Here's the drawing with two shaded views (mm, measured from the low corner). I have some questions. A direction names the side the tool comes from. Coordinates: 2 decimals unless noted, no trailing zeros. Order: outer loops, then holes, each group sorted by start corner. A loop starts at its lowest first (then second) coordinate and runs counter-clockwise, first axis right, second up. Notation, with made-up numbers: (-11.75, 23.25) -> (46.25, 23.25) arc R13 ccw to (46.25, 28.25) -> close; hole circle Ø8 at (86, -10.5). An arc over 180 degrees is marked (long way). Answer in a Markdown table with one row per item. Add a question column.
1. On a 3-axis mill with a long thin cutter (end or side, diameter ignored), from which of +Z, -Z, +X, -X, +Y, -Y can I reach the whole of each face in a straight line? I mean the marked faces 1 and 2. Say none if no direction works.
2. Imagine slicing it at D-D on y = 17. Write out the boundary of the cut face in (x, z).
3. Imagine slicing it at A-A on y = 10. Write out the boundary of the cut face in (x, z), plus the area to 3 significant figures.
4. Imagine slicing it at B-B on x = 10. Write out the boundary of the cut face in (y, z), plus the area to 3 significant figures.
5. We'd pull the mould along X, two halves only. Please class the marked faces 3, 4, 5 and 6: pulls with the +X half, pulls with the -X half, needs draft (parallel to the pull), parting line crosses it, or undercut.
6. Imagine slicing it at C-C on z = 7. Write out the boundary of the cut face in (x, y).
7. Will this pin go through, and if not, where does the flat tip stop? pin 1 (1 mm diameter, centred on y = 13, z = 10.5, fed in from +X).
8. If I drill on line 1 along Y through (x, z) = (10, 1.25); line 2 along Y through (x, z) = (0.95, 7); line 3 along X through (y, z) = (13.5, 5.75), over which ranges is the centre line in solid material (lowest first)? Write a range as [from, to].
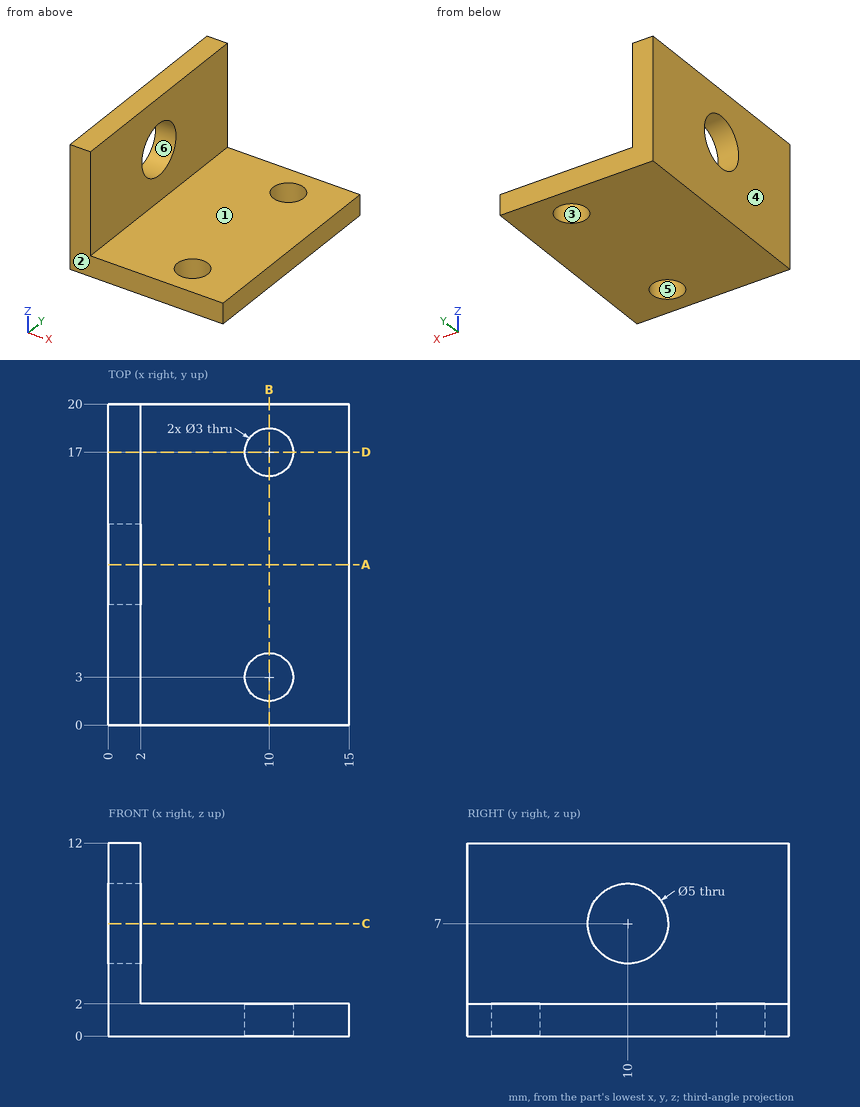
Answers follow:
| question | item | result |
|---|---|---|
| 1 | face 1 | +Z, +X, +Y, -Y |
| 1 | face 2 | +Z, -Z, +X, -X, -Y |
| 2 | outline | (0, 0) -> (8.5, 0) -> (8.5, 2) -> (2, 2) -> (2, 12) -> (0, 12) -> close; (11.5, 0) -> (15, 0) -> (15, 2) -> (11.5, 2) -> close |
| 3 | outline | (0, 0) -> (15, 0) -> (15, 2) -> (2, 2) -> (2, 4.5) -> (0, 4.5) -> close; (0, 9.5) -> (2, 9.5) -> (2, 12) -> (0, 12) -> close |
| 3 | area | 40.0 mm² |
| 4 | outline | (0, 0) -> (1.5, 0) -> (1.5, 2) -> (0, 2) -> close; (4.5, 0) -> (15.5, 0) -> (15.5, 2) -> (4.5, 2) -> close; (18.5, 0) -> (20, 0) -> (20, 2) -> (18.5, 2) -> close |
| 4 | area | 28.0 mm² |
| 5 | face 3 | undercut |
| 5 | face 4 | pulls with the -X half |
| 5 | face 5 | undercut |
| 5 | face 6 | needs draft |
| 6 | outline | (0, 0) -> (2, 0) -> (2, 7.5) -> (0, 7.5) -> close; (0, 12.5) -> (2, 12.5) -> (2, 20) -> (0, 20) -> close |
| 7 | pin 1 | stops at x = 2 |
| 8 | line 1 | y = [0, 1.5], [4.5, 15.5], [18.5, 20] |
| 8 | line 2 | y = [0, 7.5], [12.5, 20] |
| 8 | line 3 | x = [0, 2] |
